Check sheet for the drawn part. Datum: minimum x, y, z corner. Units: mm. Round coordinates to 2 decimals unless told otherwise and drop trailing zeros. Loops run counter-clockwise (first coordinate to the right, second up) from the corner with the lowest first, then second, coordinate; pieces in that order, holes last.
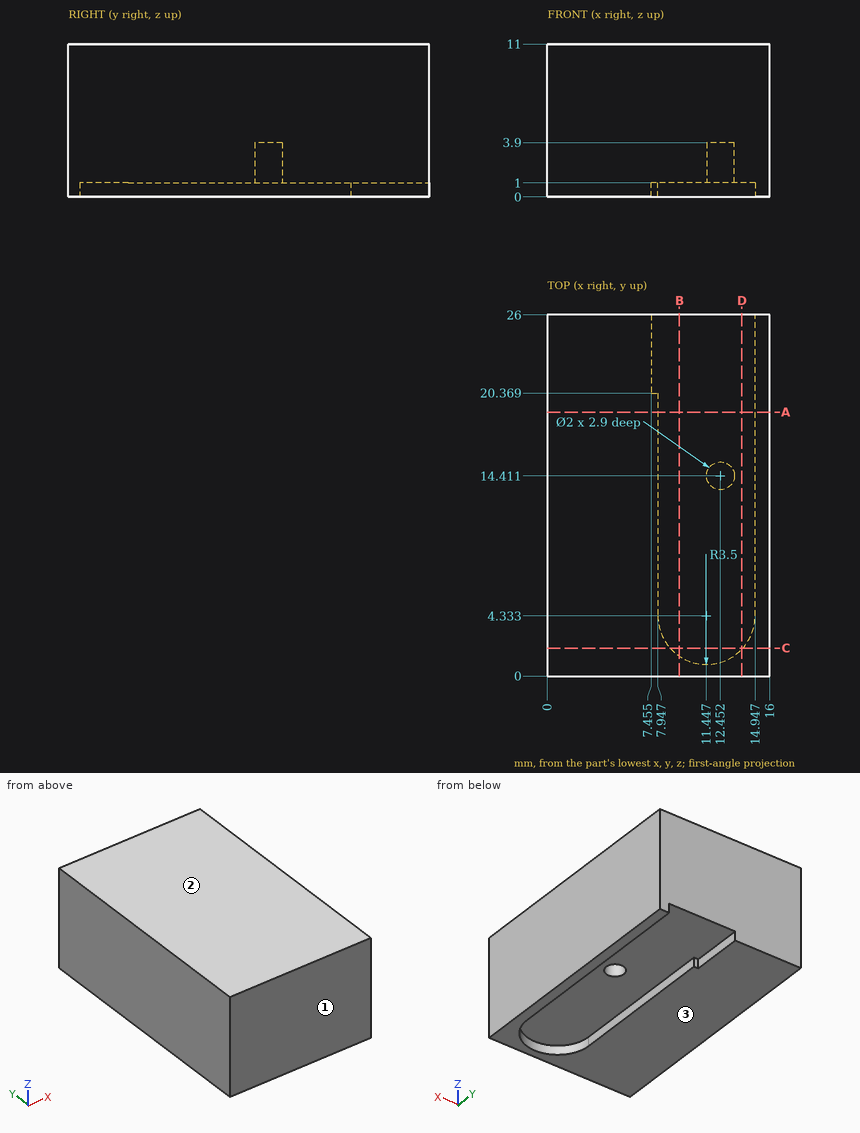
1. Scan lines: L1, parallel to X at y = 12, z = 0.5; L2, parallel to Z at x = 8.25, y = 17.5; L3, parallel to Y at x = 11.75, z = 1.75. Record each from-to range of solid material in increasing order.
2. Section check B-B (x = 9.5). Enter the section's corners in (y, z).
3. Section check A-A (y = 19). Enter the section's corners in (x, z).
4. Section check C-C (y = 2). Enter the section's corners in (x, z), then the cut area to 3 significant figures.
5. Gauge pin test, flat ends, axial feed: P1, Ø1, axis at x = 9, y = 21, coming from the -Z side; P2, Ø0.6, axis at x = 13, y = 14.5, coming from the -Z side. Record the tip position at first contact, or that the pin passes through.
6. Section check D-D (x = 14). Enter the section's corners in (y, z), then the cut area to 3 significant figures.
7. Release check for a two-part mould opening along Z. For the marked faces 1, 2 and 3 record: released by +Z, released by -Z, zero draft, split by the parting line, or undercut.
Taken from the geometry:
1. L1: x = 0 to 7.95, 14.95 to 16
1. L2: z = 1 to 11
1. L3: y = 0 to 13.7, 15.12 to 26
2. outline: (0, 0) - (1.42, 0) - (1.42, 1) - (26, 1) - (26, 11) - (0, 11) - close
3. outline: (0, 0) - (7.95, 0) - (7.95, 1) - (14.95, 1) - (14.95, 0) - (16, 0) - (16, 11) - (0, 11) - close
4. outline: (0, 0) - (8.84, 0) - (8.84, 1) - (14.06, 1) - (14.06, 0) - (16, 0) - (16, 11) - (0, 11) - close
4. area: 171 mm2
5. P1: stops at z = 1
5. P2: stops at z = 3.9
6. outline: (0, 0) - (1.94, 0) - (1.94, 1) - (26, 1) - (26, 11) - (0, 11) - close
6. area: 262 mm2
7. face 1: zero draft
7. face 2: released by +Z
7. face 3: released by -Z
